Autodesk Inventor part; units mm, degrees
sketch "Sketch1" plane through (0, 0, 0) normal (0, 0, 1) x (1, 0, 0)
  line L0 (0, 2.8582) -> (0, -2.8582) construction
  line L1 (-5.7775, 0) -> (5.7775, 0) construction
  circle A0 centre (0, 0) radius 35.629
  circle A1 centre (0, 0) radius 4
  line L2 (0, 4) -> (0, 7)
  line L3 (0, 7) -> (0, 21)
  line L4 (0, 21) -> (5, 21)
  line L5 (5, 21) -> (8, 21)
  line L6 (8, 21) -> (0, 7)
  line L7 (0, 21) -> (-8, 21)
  line L8 (-8, 21) -> (0, 7)
  line L9 (0, -4) -> (0, -7)
  line L10 (0, -7) -> (0, -21)
  line L11 (0, -21) -> (8, -21)
  line L12 (8, -21) -> (0, -7)
  line L13 (0, -21) -> (-8, -21)
  line L14 (-8, -21) -> (0, -7)
  line L15 (0, 0) -> (2.5981, 1.5)
  line L16 (0, 0) -> (3, 0) construction
  line L17 (2.5981, 1.5) -> (3.4641, 2)
  line L18 (3.4641, 2) -> (6.0622, 3.5)
  line L19 (6.0622, 3.5) -> (18.1865, 10.5)
  line L20 (18.1865, 10.5) -> (14.1865, 17.4282)
  line L21 (14.1865, 17.4282) -> (6.0622, 3.5)
  line L22 (18.1865, 10.5) -> (22.1865, 3.5718)
  line L23 (22.1865, 3.5718) -> (6.0622, 3.5)
  line L24 (0, 0) -> (8, 0) construction
  line L25 (0, 0) -> (3.4641, -2)
  line L26 (0, 0) -> (4, 0) construction
  line L27 (3.4641, -2) -> (6.0622, -3.5)
  line L28 (6.0622, -3.5) -> (18.1865, -10.5)
  line L29 (18.1865, -10.5) -> (14.1865, -17.4282)
  line L30 (14.1865, -17.4282) -> (6.0934, -3.518)
  line L31 (18.1865, -10.5) -> (22.0919, -3.518)
  line L32 (22.0919, -3.518) -> (6.0934, -3.518)
  line L33 (0, 0) -> (-2.5981, 1.5)
  line L34 (0, 0) -> (3, 0) construction
  line L35 (-2.5981, 1.5) -> (-3.4641, 2)
  line L36 (-3.4641, 2) -> (-6.0622, 3.5)
  line L37 (-6.0622, 3.5) -> (-18.1865, 10.5)
  line L38 (-18.1865, 10.5) -> (-14.1865, 17.4282)
  line L39 (-14.1865, 17.4282) -> (-6.0622, 3.5)
  line L40 (-18.1865, 10.5) -> (-22.1865, 3.5718)
  line L41 (-22.1865, 3.5718) -> (-6.0622, 3.5)
  line L42 (0, 0) -> (-6.0622, -3.5)
  line L43 (0, 0) -> (7, 0) construction
  line L44 (-6.0622, -3.5) -> (-18.1865, -10.5)
  line L45 (-18.1865, -10.5) -> (-14.1865, -17.4282)
  line L46 (-14.1865, -17.4282) -> (-6.0622, -3.5)
  line L47 (-18.1865, -10.5) -> (-22.1865, -3.5718)
  line L48 (-22.1865, -3.5718) -> (-6.0622, -3.5)
  dimension "d0" = 71.258
  dimension "d1" = 8
  dimension "d2" = 3
  dimension "d3" = 14
  dimension "d4" = 5
  dimension "d5" = 3
  dimension "d6" = 8
  dimension "d7" = 3
  dimension "d8" = 14
  dimension "d9" = 8
  dimension "d10" = 8
  dimension "d11" = 3
  dimension "d12" = 30
  dimension "d13" = 3
  dimension "d14" = 14
  dimension "d15" = 8
  dimension "d16" = 8
  dimension "d19" = 4
  dimension "d20" = 30
  dimension "d21" = 3
  dimension "d22" = 14
  dimension "d23" = 8
  dimension "d24" = 8
  dimension "d25" = 3
  dimension "d26" = 150
  dimension "d27" = 1
  dimension "d28" = 180
  dimension "d29" = 3
  dimension "d30" = 180
  dimension "d31" = 180
  dimension "d32" = 8
  dimension "d33" = 8
  dimension "d34" = 7
  dimension "d35" = 150
  dimension "d36" = 14
  dimension "d37" = 180
  dimension "d38" = 8
  dimension "d39" = 8
extrude "Extrusion1" add sketch "Sketch1" along normal blind 2
fillet "Fillet1" radius 2 18 edges at (14.1865, 17.4282, 1) (22.1865, 3.5718, 1) (6.0622, 3.5, 1) (22.0919, -3.518, 1) (14.1865, -17.4282, 1) (6.0934, -3.518, 1) (0, 7, 1) (-8, 21, 1) (8, 21, 1) (-6.0622, 3.5, 1) (-22.1865, 3.5718, 1) (-14.1865, 17.4282, 1) (-6.0622, -3.5, 1) (-14.1865, -17.4282, 1) (-22.1865, -3.5718, 1) (-8, -21, 1) (0, -7, 1) (8, -21, 1)
sketch "Sketch2" plane through (0, 0, 2) normal (0, 0, 1) x (1, 0, 0)
  circle A0 centre (0, 0) radius 3.05
  circle A1 centre (0, 0) radius 5
  dimension "d43" = 6.1
  dimension "d49" = 10
extrude "Extrusion2" add sketch "Sketch2" against normal blind 2
chamfer "Chamfer1" distance 1 angle 45 1 edges at (-35.629, 0, 2)
properties part number "Wiel hout x 20mm" material "S235"
Read the model definition and answer for the solid it produces. Units are mm, in the model's axes. Round coordinates to 2 decimals unless told otherwise and drop trailing zeros. Loops run counter-clockwise (first coordinate to the right, second up) from the corner with the lowest first, then second, coordinate; pieces in that order, holes last.
Q1. Section A-A on y = 0 is taken. Write down the section's boundary in (x, z), and give its area (3 significant figures).
Q2. Section B-B on x = 0 is taken. Write down the section's boundary in (y, z), and give its area (3 significant figures).
Q3. Determine the mould class of faces 1 (the face through (-14.153, 15.443, 1.014)), 2 (the face through (7, 0, 0)) for opening direction X: released by +X, released by -X, zero draft, split by the parting line, or undercut.
Q4. Section C-C on z = 0.55 is taken. Give the number of separate pieces and of enclosed holes in the cut face, and give its area (3 significant figures).
Q5. Each of these flat-tipped pins is pushed along its axis until it touches: pin 1 (0.6 mm diameter, centred on x = -1, z = 1.5, fed in from +Y) (3 decimals); pin 2 (1 mm diameter, centred on x = 14, z = 0.5, fed in from -Y); pin 3 (1 mm diameter, centred on y = -12, z = 1.5, fed in from +X). Where does it stop, or does it pass through?
Q6. Consider probe 1 along Y at (x, z) = (0, 1); probe 2 along Y at (x, z) = (2, 1.4); probe 3 along Y at (x, z) = (-15, 1). Determine where each line is inside the solid, lowest interval first.
Output:
1. outline: (-35.63, 0) - (-3.05, 0) - (-3.05, 2) - (-34.63, 2) - (-35.63, 1) - close; (3.05, 0) - (35.63, 0) - (35.63, 1) - (34.63, 2) - (3.05, 2) - close
1. area: 129 mm2
2. outline: (-35.63, 0) - (-21, 0) - (-21, 2) - (-34.63, 2) - (-35.63, 1) - close; (-9.03, 0) - (-3.05, 0) - (-3.05, 2) - (-9.03, 2) - close; (3.05, 0) - (9.03, 0) - (9.03, 2) - (3.05, 2) - close; (21, 0) - (35.63, 0) - (35.63, 1) - (34.63, 2) - (21, 2) - close
2. area: 81.4 mm2
3. face 1: undercut
3. face 2: zero draft
4. separate pieces: 1
4. enclosed holes: 7
4. area: 3,340 mm2
5. pin 1: stops at y = 35.415
5. pin 2: stops at y = -32.97
5. pin 3: stops at x = 33.58
6. probe 1: y = -35.63 to -21, -9.03 to -3.05, 3.05 to 9.03, 21 to 35.63
6. probe 2: y = -35.17 to -21, -10.5 to -2.3, 2.3 to 10.5, 21 to 35.17
6. probe 3: y = -32.32 to -15.27, -3.54 to 3.54, 15.27 to 32.32
